from build123d import *

# Parameters (mm, degrees)
F0_R     = 12.5
F1_DEPTH = 105
F3_DEPTH = 67
F4_R     = 3
F6_D     = 4
F6_DEPTH = 20
F6_TIP   = 1.2017212381
F7_D     = 4
F7_DEPTH = 20
F7_START = 11
F7_TIP   = 1.2017212381
F8_R     = 1


with BuildPart() as f1:
    # F0 (on Top) → F1 (new body)
    with BuildSketch(Plane.XY):
        Circle(F0_R)
    extrude(amount=F1_DEPTH)

    # F2 (on face) → F3 (join)
    with BuildSketch(Plane.XY.offset(105)):
        with BuildLine():
            Line((11.2334422785, -5.4826795069), (-11.2334422785, -5.4826795069))
            ThreePointArc((-11.2334422785, -5.4826795069), (0, -12.5), (11.2334422785, -5.4826795069))
        make_face()
        with BuildLine():
            ThreePointArc((11.2164688996, 5.5173204931), (0, 12.5), (-11.2164688996, 5.5173204931))
            Line((-11.2164688996, 5.5173204931), (11.2164688996, 5.5173204931))
        make_face()
    extrude(amount=F3_DEPTH)

    # F4
    f4_edges = [f1.edges().sort_by_distance(p)[0] for p in [
        (-12.5, 0, 0),
    ]]
    fillet(f4_edges, radius=F4_R)

    # F6 (one way)
    with BuildSketch(Plane.XZ.offset(-5.5173204931)):
        with Locations((0, 162)):
            Circle(F6_D / 2)
    extrude(amount=-F6_DEPTH, mode=Mode.SUBTRACT)
    with Locations(Plane.XZ.offset(-5.5173204931)):
        with Locations((0, 162)):
            with Locations((0, 0, -(F6_DEPTH + F6_TIP / 2))):  # 118° drill point
                Cone(0, F6_D / 2, F6_TIP, mode=Mode.SUBTRACT)

    # F7
    # its depths count from where the whole tool has entered the part; down to there all is cleared
    with Locations(Plane(origin=(0, 5.5173204931, 0), x_dir=(1, 0, 0), z_dir=(0, 1, 0)).offset(-F7_START)):
        with Locations((0, -162)):
            Hole(F7_D / 2, depth=F7_DEPTH)
            with Locations((0, 0, -(F7_DEPTH + F7_TIP / 2))):  # 118° drill point
                Cone(0, F7_D / 2, F7_TIP, mode=Mode.SUBTRACT)

    # F8
    f8_edges = [f1.edges().sort_by_distance(p)[0] for p in [
        (0, 12.5, 172),
        (0, -12.5, 172),
    ]]
    fillet(f8_edges, radius=F8_R)


solid = f1.part
Could you check a few things on this model? Use its own coordinates, in mm. A direction names the side the tool comes from. Round coordinates to 2 decimals unless told otherwise and drop trailing zeros. Write each loop counter-clockwise with the first axis right and the second up, starting at its lowest first coordinate (ties: lowest second). Pieces come first, ordered by that corner, then holes. Notation, with made-up numbers: (-3, 43) - (55, 43) arc R21 cw to (55, 70) - close; hole circle Ø2 at (-9, -22.5). An arc over 180 degrees is marked (long way). Use a Markdown table: item, result.
Q1. For pin 1 (1 mm diameter, centred on x = 4.5, z = 140, fed in from -Y); pin 2 (6 mm diameter, centred on x = -6, z = 34.5, fed in from +Y); pin 3 (1 mm diameter, centred on x = -1, z = 71.5, fed in from -Y), each with a flat end and sliding along its axis, tell me the tip position at first contact or that it passes through.
Output values:
| item | result |
|---|---|
| pin 1 | y = -11.84 |
| pin 2 | y = 12.13 |
| pin 3 | y = -12.49 |
Q2. I want a section at C-C (z = 162). List the corners of the cut face in (x, y) for me, plus the area to 3 significant figures.
Output values:
| item | result |
|---|---|
| outline | (-11.23, -5.48) arc R12.5 ccw to (-2, -12.34) - (-2, -5.48) - close; (-11.22, 5.52) - (-2, 5.52) - (-2, 12.34) arc R12.5 ccw to start; (2, -12.34) arc R12.5 ccw to (11.23, -5.48) - (2, -5.48) - close; (2, 5.52) - (11.22, 5.52) arc R12.5 ccw to (2, 12.34) - close |
| area | 169 mm2 |
Q3. I want a section at A-A (x = 0). List the corners of the cut face in (y, z) for me, plus the area to 3 significant figures.
Output values:
| item | result |
|---|---|
| outline | (-12.5, 3) arc R3 ccw to (-9.5, 0) - (9.5, 0) arc R3 ccw to (12.5, 3) - (12.5, 160) - (5.52, 160) - (5.52, 105) - (-5.48, 105) - (-5.48, 160) - (-12.5, 160) - close; (-12.5, 164) - (-5.48, 164) - (-5.48, 172) - (-11.5, 172) arc R1 ccw to (-12.5, 171) - close; (5.52, 164) - (12.5, 164) - (12.5, 171) arc R1 ccw to (11.5, 172) - (5.52, 172) - close |
| area | 3,500 mm2 |
Q4. I want a section at D-D (z = 131). List the corners of the cut face in (x, y) for me.
Output values:
| item | result |
|---|---|
| outline | (-11.23, -5.48) arc R12.5 ccw to (11.23, -5.48) - close; (-11.22, 5.52) - (11.22, 5.52) arc R12.5 ccw to start |
Q5. Please list where these lines run through material, in increasing order: L1, parallel to Z at x = 0, y = 8; L2, parallel to X at y = -10.75, z = 162; L3, parallel to X at y = 8.5, z = 162.
Output values:
| item | result |
|---|---|
| L1 | 0 to 160, 164 to 172 |
| L2 | -6.38 to -2, 2 to 6.38 |
| L3 | -9.17 to -2, 2 to 9.17 |
Q6. Thinking about a two-plate mould opening in Y: for faces 1 (the flat face through (0, 0, 105)), 2 (the flat face through (0, 8, 172)), which applies, released by +Y, released by -Y, zero draft, split by the parting line, or undercut?
Output values:
| item | result |
|---|---|
| face 1 | undercut |
| face 2 | zero draft |
Q7. For faces 3 (the cylindrical face through (-0.923, -9.043, 163.774)), 4 (the flat face through (0, 5.517, 138)), which set-ups out of +Z, -Z, +X, -X, +Y, -Y let a thin tool reach every point of the face, with its end or its side?
Output values:
| item | result |
|---|---|
| face 3 | +Y, -Y |
| face 4 | +Z, +X, -X |
Q8. I want a section at B-B (y = 0). List the corners of the cut face in (x, z) for me, plus the area to 3 significant figures.
Output values:
| item | result |
|---|---|
| outline | (-12.5, 3) arc R3 ccw to (-9.5, 0) - (9.5, 0) arc R3 ccw to (12.5, 3) - (12.5, 105) - (-12.5, 105) - close |
| area | 2,620 mm2 |
